The model under review builds one solid part; all positions refer to its coordinate system, in mm. A direction names the side the tool comes from. Round coordinates to 2 decimals unless told otherwise and drop trailing zeros. Loops run counter-clockwise (first coordinate to the right, second up) from the corner with the lowest first, then second, coordinate; pieces in that order, holes last. Notation, with made-up numbers: M 75.25,-1.5 L 112.25,-1.5 A4 ccw 112.25,4.5 Z; hole C 48,-19.5 d1. An arc over 180 degrees is marked long. One line per question, with ' | ' between items.
Solid Edge part; units mm, degrees
sketch "Sketch1" plane through (0, 0, 0) normal (0, -1, 0) x (1, 0, 0)
  line L0 (-45, -40) -> (45, -40)
  line L1 (45, -40) -> (45, 40)
  line L2 (45, 40) -> (-45, 40)
  line L3 (-45, 40) -> (-45, -40)
  dimension "D1" = 45
  dimension "D2" = 45
extrude "Protrusion1" add sketch "Sketch1" against normal blind 10
sketch "Sketch2" plane through (0, 0, 0) normal (0, -1, 0) x (1, 0, 0)
  circle A0 centre (-40, 30) radius 1.4
  circle A1 centre (-40, -30) radius 1.4
  circle A2 centre (40, -30) radius 1.4
  circle A3 centre (40, 30) radius 1.4
  dimension "D1" = 40
  dimension "D2" = 40
extrude "Cutout1" cut sketch "Sketch2" against normal through all
sketch "Sketch3" plane through (0, 0, 0) normal (0, -1, 0) x (1, 0, 0)
  circle A0 centre (-21, 16) radius 4
  circle A1 centre (-21, -16) radius 4
  circle A2 centre (21, -16) radius 4
  circle A3 centre (21, 16) radius 4
extrude "Extrusionsausschnitt_2" cut sketch "Sketch3" against normal blind 5
sketch "Sketch4" plane through (0, 0, 0) normal (0, -1, 0) x (1, 0, 0)
  circle A0 centre (-21, 16) radius 1.75
  circle A1 centre (-21, -16) radius 1.75
  circle A2 centre (21, -16) radius 1.75
  circle A3 centre (21, 16) radius 1.75
extrude "Cutout2" cut sketch "Sketch4" against normal through all
fillet "Verrundung_1" radius 4 4 edges at (-45, 5, 40) (45, 5, 40) (45, 5, -40) (-45, 5, -40)
chamfer "Fase_1" distance 0.5 angle 60 4 edges at (38.6, 0, 30) (-41.4, 0, 30) (-41.4, 0, -30) (38.6, 0, -30) measured on face at (-29.1, 0, 27.4667)
chamfer "Fase_2" distance 0.5 angle 60 4 edges at (-40, 10, 31.4) (40, 10, 31.4) (40, 10, -28.6) (-40, 10, -28.6) measured on face at (-29.1, 10, 27.4667)
chamfer "Fase_3" distance 0.5 angle 60 4 edges at (-21, 10, 17.75) (21, 10, 17.75) (-21, 10, -14.25) (21, 10, -14.25) measured on face at (-29.1, 10, 27.4667)
chamfer "Fase_4" distance 0.5 angle 60 4 edges at (-21, 5, 14.25) (-21, 5, -17.75) (21, 5, 14.25) (21, 5, -17.75) measured on face at (-23.5867, 5, 18.7467) measured on face at (18.4133, 5, 18.7467) measured on face at (-23.5867, 5, -13.2533) measured on face at (18.4133, 5, -13.2533)
sketch "Sketch5" plane through (0, 10, 0) normal (0, 1, 0) x (1, 0, 0)
  line L0 (-45, 11) -> (-37, 11)
  line L1 (-37, 11) -> (-37, 18)
  line L2 (-37, 18) -> (-45, 18)
  line L3 (-45, 18) -> (-45, 11)
  dimension "D1" = 45
  dimension "D2" = 45
extrude "Extrusionsausprägung_2" add sketch "Sketch5" along normal blind 14
mirror "Mirror1" about plane through (0, 0, 0) normal (0, 0, 1) of "Extrusionsausprägung_2"
mirror "Mirror2" about plane through (0, 0, 0) normal (1, 0, 0) of "Extrusionsausprägung_2", "Mirror1"
properties material "Nylon, allgemein"
1) Insertion check: P1, Ø6.5, axis at x = 21, z = 16, coming from the +Y side; P2, Ø2.5, axis at x = 40.5, y = 20, coming from the -Z side; P3, Ø2.5, axis at x = 41.5, y = 20.5, coming from the +Z side. Each pin has a flat end and moves straight along its axis. Give the tip position at first contact, or say it passes through.
Output values:
P1: stops at y = 10 | P2: stops at z = -18 | P3: stops at z = 18
2) For line 1 (Z direction, x = 21, y = 2.2); line 2 (X direction, y = 10.5, z = -17); line 3 (Z direction, x = 21, y = 7.1), list the stretches that pass through material, from the lowest coordinate up.
Output values:
line 1: z = -40 to -20, -12 to 12, 20 to 40 | line 2: x = -45 to -37, 37 to 45 | line 3: z = -40 to -17.75, -14.25 to 14.25, 17.75 to 40
3) Add section C-C on y = 15.75. State the section outline as (x, z) points.
Output values:
outline: M -45,-18 L -37,-18 L -37,-11 L -45,-11 Z; M -45,11 L -37,11 L -37,18 L -45,18 Z; M 37,-18 L 45,-18 L 45,-11 L 37,-11 Z; M 37,11 L 45,11 L 45,18 L 37,18 Z
4) Mouldability with a two-part tool opening along Z and no side actions: class faces 1 (the flat face through (-41, 17, 11)), 2 (the cylindrical face through (18.05, 2.46, -13.3)), 3 (the flat face through (41, 24, 15)) as +Z half, -Z half, draft (parallel to the pull), parting line (faces both ways), or undercut.
Output values:
face 1: undercut | face 2: undercut | face 3: draft
5) Machinability: for faces 4 (the flat face through (37, 17, 14)), 5 (the flat face through (19, 5, -18)), 6 (the cylindrical face through (-39.25, 4.94, -28.82)), which of the approach directions +Z, -Z, +X, -X, +Y, -Y give a long, thin tool a straight path to every point of the face, cutting with its end or side? Answer none if there is none.
Output values:
face 4: +Z, -Z, +Y | face 5: -Y | face 6: +Y, -Y
6) Add section A-A on x = 21. State the section outline as (y, z) points, then the cut area to 3 significant figures.
Output values:
outline: M 0,-40 L 10,-40 L 10,-18.25 L 9.13,-17.75 L 5.87,-17.75 L 5,-18.25 L 5,-20 L 0,-20 Z; M 0,-12 L 5,-12 L 5,-13.75 L 5.87,-14.25 L 9.13,-14.25 L 10,-13.75 L 10,13.75 L 9.13,14.25 L 5.87,14.25 L 5,13.75 L 5,12 L 0,12 Z; M 0,20 L 5,20 L 5,18.25 L 5.87,17.75 L 9.13,17.75 L 10,18.25 L 10,40 L 0,40 Z | area: 683 mm²
7) Add section B-B on z = -16. State how many separate pieces and enclosed holes the cut face has, then the cut area to 3 significant figures.
Output values:
separate pieces: 3 | enclosed holes: 0 | area: 1,010 mm²
